from build123d import *

# Parameters (mm, degrees)
BOSS_EXTRUDE1_DEPTH = 6.2
BOSS_EXTRUDE2_DEPTH = 21
CHAMFER1_SIZE       = 5
CHAMFER1_SIZE2      = 28.356409098
CUT_EXTRUDE1_REACH  = 73.991
CHAMFER2_SIZE       = 1
CHAMFER2_SIZE2      = 9.514364454
CHAMFER3_SIZE       = 2
CUT_EXTRUDE2_REACH  = 78.94
CUT_EXTRUDE3_START  = -3.468867
CUT_EXTRUDE3_DEPTH  = 3.468867
BOSS_EXTRUDE3_DEPTH = 6.2
CUT_EXTRUDE4_REACH  = 78.94


with BuildPart() as part:
    # Sketch1 → Boss-Extrude1 (new body)
    with BuildSketch(Plane.XY):
        with BuildLine():
            Line((-28, 0), (0, 0))
            Line((0, 0), (0, 10))
            Line((0, 10), (-7.1, 10))
            ThreePointArc((-7.1, 10), (-14.171067812, 12.928932188), (-17.1, 20))
            Line((-17.1, 20), (-17.1, 51))
            Line((-17.1, 51), (-20.1, 51))
            Line((-20.1, 51), (-20.1, 6))
            Line((-20.1, 6), (-24, 6))
            Line((-24, 6), (-24, 50))
            Line((-24, 50), (-28, 50))
            Line((-28, 50), (-28, 0))
        make_face()
    extrude(amount=BOSS_EXTRUDE1_DEPTH)

    # Sketch2 → Boss-Extrude2 (add)
    with BuildSketch(Plane.XZ):
        Polygon((0, 6.2), (0, 10.4), (11, 10.4), (11, 42.4), (-24.1, 42.4), (-24.1, 10.4), (-13.1, 10.4), (-13.1, 6.2), align=None)
    extrude(amount=-BOSS_EXTRUDE2_DEPTH)

    # Chamfer1
    chamfer1_edges = [part.edges().sort_by_distance(p)[0] for p in [
        (-6.55, 0, 42.4),
    ]]
    chamfer1_side = [part.faces().sort_by_distance(p)[0] for p in [
        (-6.55, 10.5, 42.4),
    ]]
    chamfer(chamfer1_edges, length=CHAMFER1_SIZE, length2=CHAMFER1_SIZE2, reference=chamfer1_side[0])

    # Sketch3 → Cut-Extrude1 (cut, up to next)
    with BuildSketch(Plane(origin=(0, 0, 0), x_dir=(0, 0, -1), z_dir=(1, 0, 0)), mode=Mode.PRIVATE) as cut_extrude1_sk1:
        Polygon((-6.2, 10), (-7.6, 10), (-10.4, 21), (-6.2, 21), align=None)
    cut_extrude1_tool1 = extrude(cut_extrude1_sk1.sketch, amount=-CUT_EXTRUDE1_REACH, mode=Mode.PRIVATE) & part.part
    add(cut_extrude1_tool1.solids().sort_by_distance((0, 16.416667, 7.716667))[0], mode=Mode.SUBTRACT)

    # Chamfer2
    chamfer2_edges = [part.edges().sort_by_distance(p)[0] for p in [
        (11, 10.5, 10.4),
    ]]
    chamfer2_side = [part.faces().sort_by_distance(p)[0] for p in [
        (11, 11.541747932, 25.62778603),
    ]]
    chamfer(chamfer2_edges, length=CHAMFER2_SIZE, length2=CHAMFER2_SIZE2, reference=chamfer2_side[0])

    # Chamfer3
    chamfer3_edges = [part.edges().sort_by_distance(p)[0] for p in [
        (-24.1, 10.5, 10.4),
    ]]
    chamfer(chamfer3_edges, length=CHAMFER3_SIZE)

    # Sketch5 → Cut-Extrude2 (cut, up to next)
    with BuildSketch(Plane(origin=(11, 0, 0), x_dir=(0, 0, -1), z_dir=(1, 0, 0)), mode=Mode.PRIVATE) as cut_extrude2_sk1:
        Polygon((-42.4, 17.8), (-13.86886709, 5), (-10.966215349, -4.108657177), (-44.036924755, 0.937700744), align=None)
    cut_extrude2_tool1 = extrude(cut_extrude2_sk1.sketch, amount=-CUT_EXTRUDE2_REACH, mode=Mode.PRIVATE) & part.part
    add(cut_extrude2_tool1.solids().sort_by_distance((11, 5.258773, 29.627692))[0], mode=Mode.SUBTRACT)

    # Sketch6 → Cut-Extrude3 (cut)
    with BuildSketch(Plane(origin=(0, 0, 10.4), x_dir=(-1, 0, 0), z_dir=(0, 0, -1)).offset(CUT_EXTRUDE3_START)):
        Polygon((13.1, 0), (24.1, 5), (37.198342989, 5), (28.62602328, -4.522208447), (-13.825974113, -5.629287686), (-20.705007466, 5), (-11, 5), (0, 0), align=None)
    extrude(amount=CUT_EXTRUDE3_DEPTH, mode=Mode.SUBTRACT)

    # Sketch7 → Boss-Extrude3 (add)
    with BuildSketch(Plane.XY.offset(6.2)):
        with BuildLine():
            Line((-16.7, 50.6), (-15.7, 50.5))
            ThreePointArc((-15.7, 50.5), (-15.462165524, 50.365875857), (-15.4, 50.1))
            ThreePointArc((-15.4, 50.1), (-15.462165524, 49.834124143), (-15.7, 49.7))
            Line((-15.7, 49.7), (-16.7, 49.6))
            ThreePointArc((-16.7, 49.6), (-16.971392676, 49.471392676), (-17.1, 49.2))
            Line((-17.1, 49.2), (-17.1, 48.9))
            ThreePointArc((-17.1, 48.9), (-16.971392676, 48.628607324), (-16.7, 48.5))
            Line((-16.7, 48.5), (-15.7, 48.4))
            ThreePointArc((-15.7, 48.4), (-15.462165524, 48.265875857), (-15.4, 48))
            ThreePointArc((-15.4, 48), (-15.462165524, 47.734124143), (-15.7, 47.6))
            Line((-15.7, 47.6), (-16.7, 47.5))
            ThreePointArc((-16.7, 47.5), (-16.971392676, 47.371392676), (-17.1, 47.1))
            Line((-17.1, 47.1), (-17.1, 46.8))
            ThreePointArc((-17.1, 46.8), (-16.971392676, 46.528607324), (-16.7, 46.4))
            Line((-16.7, 46.4), (-15.7, 46.3))
            ThreePointArc((-15.7, 46.3), (-15.462165524, 46.165875857), (-15.4, 45.9))
            ThreePointArc((-15.4, 45.9), (-15.462165524, 45.634124143), (-15.7, 45.5))
            Line((-15.7, 45.5), (-16.7, 45.4))
            ThreePointArc((-16.7, 45.4), (-16.971392676, 45.271392676), (-17.1, 45))
            Line((-17.1, 45), (-17.1, 44.7))
            ThreePointArc((-17.1, 44.7), (-16.971392676, 44.428607324), (-16.7, 44.3))
            Line((-16.7, 44.3), (-15.7, 44.2))
            ThreePointArc((-15.7, 44.2), (-15.462165524, 44.065875857), (-15.4, 43.8))
            ThreePointArc((-15.4, 43.8), (-15.462165524, 43.534124143), (-15.7, 43.4))
            Line((-15.7, 43.4), (-16.7, 43.3))
            ThreePointArc((-16.7, 43.3), (-16.971392676, 43.171392676), (-17.1, 42.9))
            Line((-17.1, 42.9), (-17.1, 42.6))
            ThreePointArc((-17.1, 42.6), (-16.971392676, 42.328607324), (-16.7, 42.2))
            Line((-16.7, 42.2), (-15.7, 42.1))
            ThreePointArc((-15.7, 42.1), (-15.462165524, 41.965875857), (-15.4, 41.7))
            ThreePointArc((-15.4, 41.7), (-15.462165524, 41.434124143), (-15.7, 41.3))
            Line((-15.7, 41.3), (-16.7, 41.2))
            ThreePointArc((-16.7, 41.2), (-16.971392676, 41.071392676), (-17.1, 40.8))
            Line((-17.1, 40.8), (-17.1, 40.5))
            ThreePointArc((-17.1, 40.5), (-16.971392676, 40.228607324), (-16.7, 40.1))
            Line((-16.7, 40.1), (-15.7, 40))
            ThreePointArc((-15.7, 40), (-15.462165524, 39.865875857), (-15.4, 39.6))
            ThreePointArc((-15.4, 39.6), (-15.462165524, 39.334124143), (-15.7, 39.2))
            Line((-15.7, 39.2), (-16.7, 39.1))
            ThreePointArc((-16.7, 39.1), (-16.971392676, 38.971392676), (-17.1, 38.7))
            Line((-17.1, 38.7), (-17.1, 38.4))
            ThreePointArc((-17.1, 38.4), (-16.971392676, 38.128607324), (-16.7, 38))
            Line((-16.7, 38), (-15.7, 37.9))
            ThreePointArc((-15.7, 37.9), (-15.462165524, 37.765875857), (-15.4, 37.5))
            ThreePointArc((-15.4, 37.5), (-15.462165524, 37.234124143), (-15.7, 37.1))
            Line((-15.7, 37.1), (-16.7, 37))
            ThreePointArc((-16.7, 37), (-16.971392676, 36.871392676), (-17.1, 36.6))
            Line((-17.1, 36.6), (-17.1, 36.3))
            ThreePointArc((-17.1, 36.3), (-16.971392676, 36.028607324), (-16.7, 35.9))
            Line((-16.7, 35.9), (-15.7, 35.8))
            ThreePointArc((-15.7, 35.8), (-15.462165524, 35.665875857), (-15.4, 35.4))
            ThreePointArc((-15.4, 35.4), (-15.462165524, 35.134124143), (-15.7, 35))
            Line((-15.7, 35), (-16.7, 34.9))
            ThreePointArc((-16.7, 34.9), (-16.971392676, 34.771392676), (-17.1, 34.5))
            Line((-17.1, 34.5), (-17.1, 34.2))
            ThreePointArc((-17.1, 34.2), (-16.971392676, 33.928607324), (-16.7, 33.8))
            Line((-16.7, 33.8), (-15.7, 33.7))
            ThreePointArc((-15.7, 33.7), (-15.462165524, 33.565875857), (-15.4, 33.3))
            ThreePointArc((-15.4, 33.3), (-15.462165524, 33.034124143), (-15.7, 32.9))
            Line((-15.7, 32.9), (-16.7, 32.8))
            ThreePointArc((-16.7, 32.8), (-16.971392676, 32.671392676), (-17.1, 32.4))
            Line((-17.1, 32.4), (-17.1, 32.1))
            ThreePointArc((-17.1, 32.1), (-16.971392676, 31.828607324), (-16.7, 31.7))
            Line((-16.7, 31.7), (-15.7, 31.6))
            ThreePointArc((-15.7, 31.6), (-15.462165524, 31.465875857), (-15.4, 31.2))
            ThreePointArc((-15.4, 31.2), (-15.462165524, 30.934124143), (-15.7, 30.8))
            Line((-15.7, 30.8), (-16.7, 30.7))
            ThreePointArc((-16.7, 30.7), (-16.971392676, 30.571392676), (-17.1, 30.3))
            Line((-17.1, 30.3), (-17.1, 30))
            ThreePointArc((-17.1, 30), (-16.971392676, 29.728607324), (-16.7, 29.6))
            Line((-16.7, 29.6), (-15.7, 29.5))
            ThreePointArc((-15.7, 29.5), (-15.462165524, 29.365875857), (-15.4, 29.1))
            ThreePointArc((-15.4, 29.1), (-15.462165524, 28.834124143), (-15.7, 28.7))
            Line((-15.7, 28.7), (-16.7, 28.6))
            ThreePointArc((-16.7, 28.6), (-16.971392676, 28.471392676), (-17.1, 28.2))
            Line((-17.1, 28.2), (-17.1, 27.9))
            ThreePointArc((-17.1, 27.9), (-16.971392676, 27.628607324), (-16.7, 27.5))
            Line((-16.7, 27.5), (-15.7, 27.4))
            ThreePointArc((-15.7, 27.4), (-15.462165524, 27.265875857), (-15.4, 27))
            ThreePointArc((-15.4, 27), (-15.462165524, 26.734124143), (-15.7, 26.6))
            Line((-15.7, 26.6), (-16.7, 26.5))
            ThreePointArc((-16.7, 26.5), (-16.971392676, 26.371392676), (-17.1, 26.1))
            Line((-17.1, 26.1), (-17.1, 25.8))
            ThreePointArc((-17.1, 25.8), (-16.971392676, 25.528607324), (-16.7, 25.4))
            Line((-16.7, 25.4), (-15.7, 25.3))
            ThreePointArc((-15.7, 25.3), (-15.462165524, 25.165875857), (-15.4, 24.9))
            ThreePointArc((-15.4, 24.9), (-15.462165524, 24.634124143), (-15.7, 24.5))
            Line((-15.7, 24.5), (-16.7, 24.4))
            ThreePointArc((-16.7, 24.4), (-16.971392676, 24.271392676), (-17.1, 24))
            Line((-17.1, 24), (-17.1, 23.7))
            ThreePointArc((-17.1, 23.7), (-16.971392676, 23.428607324), (-16.7, 23.3))
            Line((-16.7, 23.3), (-15.7, 23.2))
            ThreePointArc((-15.7, 23.2), (-15.462165524, 23.065875857), (-15.4, 22.8))
            ThreePointArc((-15.4, 22.8), (-15.462165524, 22.534124143), (-15.7, 22.4))
            Line((-15.7, 22.4), (-16.7, 22.3))
            ThreePointArc((-16.7, 22.3), (-16.971392676, 22.171392676), (-17.1, 21.9))
            Line((-17.1, 21.9), (-17.1, 21.6))
            ThreePointArc((-17.1, 21.6), (-16.971392676, 21.328607324), (-16.7, 21.2))
            Line((-16.7, 21.2), (-15.7, 21.1))
            ThreePointArc((-15.7, 21.1), (-15.462165524, 20.965875857), (-15.4, 20.7))
            ThreePointArc((-15.4, 20.7), (-15.462165524, 20.434124143), (-15.7, 20.3))
            Line((-15.7, 20.3), (-16.7, 20.2))
            ThreePointArc((-16.7, 20.2), (-16.971392676, 20.071392676), (-17.1, 19.8))
            Line((-17.1, 19.8), (-17.1, 19.5))
            Line((-17.1, 19.5), (-18.637373825, 21.126261745))
            Line((-18.637373825, 21.126261745), (-18.815, 46.4))
            Line((-18.815, 46.4), (-17.1, 51))
            ThreePointArc((-17.1, 51), (-16.971392676, 50.728607324), (-16.7, 50.6))
        make_face()
    extrude(amount=-BOSS_EXTRUDE3_DEPTH)

    # Sketch8 → Cut-Extrude4 (cut, up to next)
    with BuildSketch(Plane(origin=(11, 0, 0), x_dir=(0, 0, -1), z_dir=(1, 0, 0)), mode=Mode.PRIVATE) as cut_extrude4_sk1:
        Polygon((-35.4, 21), (-27.4, 17), (-19.4, 21), align=None)
    cut_extrude4_tool1 = extrude(cut_extrude4_sk1.sketch, amount=-CUT_EXTRUDE4_REACH, mode=Mode.PRIVATE) & part.part
    add(cut_extrude4_tool1.solids().sort_by_distance((11, 19.666667, 27.4))[0], mode=Mode.SUBTRACT)


solid = part.part
Model file for the job. Use its own axes, mm. A direction names the side the tool comes from. Round coordinates to 2 decimals unless told otherwise and drop trailing zeros. Order: outer loops, then holes, each group sorted by start corner. A loop starts at its lowest first (then second) coordinate and runs counter-clockwise, first axis right, second up. Notation, with made-up numbers: M 86,16.5 L 145,16.5 A17 cw 145,45.5 Z; hole C 2.25,-9 d1. An arc over 180 degrees is marked long. Write each question's results on one line, items separated by ' | '. Start each with the question number.
(1) Saw through at C-C, the plane z = 31.5. Give the cut face in (x, y), then the cut area to 3 significant figures.
(2) Probe probe 1 along X at (y, z) = (17, 27.5); probe 2 along Z at (x, y) = (-26, 35.5); probe 3 along X at (y, z) = (42.5, 5). List the from-to ranges inside material, lowest first. Write a range as from..to.
(3) Drop flat-ended pins along their axis: pin 1 (2 mm diameter, centred on x = -1, z = 37.5, fed in from +Y); pin 2 (1.2 mm diameter, centred on x = 1, y = 14.5, fed in from -Z); pin 3 (8 mm diameter, centred on y = 15, z = 28.5, fed in from -X); pin 4 (4.5 mm diameter, centred on x = -22, z = 4.5, fed in from +Y). Give the stop position or say it passes through.
(4) Saw through at A-A, the plane x = -3. Give the cut face in (y, z), then the cut area to 3 significant figures.
(5) Two-plate mould, pull along Y, no slides. Class faces 1 (the face through (0, 6, 6)), 2 (the face through (-14.03, 12.79, 3.06)), 3 (the face through (-6.46, 15.42, 8.98)): pulls with the +Y half, pulls with the -Y half, needs draft (parallel to the pull), parting line crosses it, or undercut.
(6) Saw through at D-D, the plane x = 5. Give the cut face in (y, z).
(7) Which spindle directions (+Z, -Z, +X, -X, +Y, -Y) get a long thin tool onto all of the face, cutting with end or side? Do faces 4 (the face through (-13.1, 8, 9)), 5 (the face through (-22, 6, 3)), 6 (the face through (1, 10, 10.4)), 7 (the face through (-24.1, 15, 24)), 8 (the face through (-6.3, 19.03, 31.46)). Say none if no direction does.
(8) Saw through at B-B, the plane x = -21. Give the cut face in (y, z), then the cut area to 3 significant figures.
Established:
1) outline: M -24.1,12.91 L 11,12.91 L 11,19.05 L -24.1,19.05 Z | area: 216 mm^2
2) probe 1: x = -24.1..11 | probe 2: z = 0..6.2 | probe 3: x = -28..-24, -20.1..-17.08
3) pin 1: stops at y = 21 | pin 2: stops at z = 10.4 | pin 3: stops at x = -24.1 | pin 4: stops at y = 51
4) outline: M 0,0 L 10,0 L 10,7.6 L 21,10.4 L 21,19.4 L 17,27.4 L 21,35.4 L 21,42.4 L 17.8,42.4 L 5,13.87 L 0,12.28 Z | area: 430 mm^2
5) face 1: needs draft | face 2: undercut | face 3: pulls with the +Y half
6) outline: M 2.27,10.77 L 21,10.77 L 21,19.4 L 17,27.4 L 21,35.4 L 21,42.4 L 17.8,42.4 L 5,13.87 L 2.27,13 Z
7) face 4: -X, +Y, -Y | face 5: -Z, +Y | face 6: -Z, +X, +Y, -Y | face 7: +Z, -X, +Y, -Y | face 8: +X, -X, +Y
8) outline: M 0,0 L 6,0 L 6,6.2 L 0,6.2 Z; M 3.59,10.4 L 21,10.4 L 21,19.4 L 17,27.4 L 21,35.4 L 21,42.4 L 17.8,42.4 L 5,13.87 L 3.59,13.42 Z | area: 339 mm^2
